Part model, mm, in its own coordinate system. Give positions to 0.01 mm unless a question says otherwise; leave off trailing zeros. Order: outer loops, then holes, each group sorted by start corner. A loop starts at its lowest first (then second) coordinate and runs counter-clockwise, first axis right, second up. Notation, with made-up numbers: M 85,-23 L 93,-23 A18 cw 93,-18 Z; hole C 59.25,9.25 d2. An arc over 180 degrees is marked long. Return JSON: item names as keys, results as strings.
from build123d import *

# Parameters (mm, degrees)
SKETCH1_W           = 49
SKETCH1_H           = 49
SKETCH1_R           = 2
BOSS_EXTRUDE1_DEPTH = 1.6
CHAMFER1_SIZE       = 5
CHAMFER2_SIZE       = 2


with BuildPart() as part:
    # Sketch1 → Boss-Extrude1 (new body)
    with BuildSketch(Plane(origin=(0, 0, 0), x_dir=(0, 1, 0), z_dir=(0, 0, 1))):
        with Locations((24.5, 24.5)):
            Rectangle(SKETCH1_W, SKETCH1_H)
        with Locations(Location((24.5, 26.5, 0), (0, 0, 270))):
            Circle(SKETCH1_R, mode=Mode.SUBTRACT)
    extrude(amount=-BOSS_EXTRUDE1_DEPTH)

    # Chamfer1
    chamfer1_edges = [part.edges().sort_by_distance(p)[0] for p in [
        (-49, 49, -0.8),
    ]]
    chamfer(chamfer1_edges, length=CHAMFER1_SIZE)

    # Chamfer2
    chamfer2_edges = [part.edges().sort_by_distance(p)[0] for p in [
        (-49, 0, -0.8),
        (0, 49, -0.8),
        (0, 0, -0.8),
    ]]
    chamfer(chamfer2_edges, length=CHAMFER2_SIZE)


solid = part.part
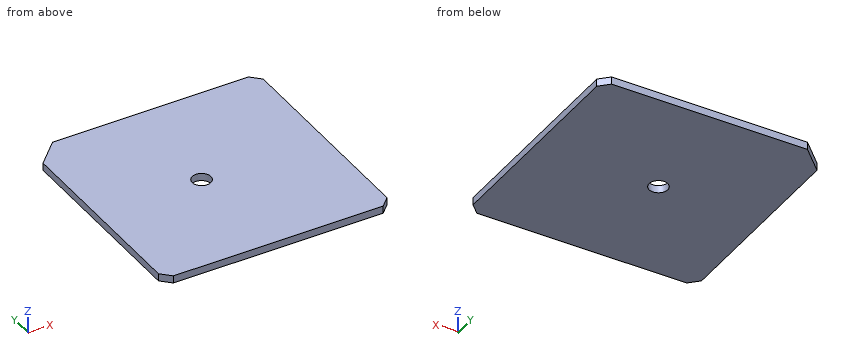
Q1. Pin check, flat tips, straight feed: pin 1 (3.5 mm diameter, centred on x = -26.5, y = 24.5, fed in from -Z); pin 2 (2 mm diameter, centred on x = -43, y = 42, fed in from +Z). Stop position of each tip, or through.
Established:
{"pin 1": "passes through", "pin 2": "stops at z = 0"}
Q2. Band-saw the part on B-B (y = 24.5). Give the cut face in (x, z).
Established:
{"outline": "M -49,-1.6 L -28.5,-1.6 L -28.5,0 L -49,0 Z; M -24.5,-1.6 L 0,-1.6 L 0,0 L -24.5,0 Z"}
Q3. Band-saw the part on A-A (x = -26.5). Give the cut face in (y, z).
Established:
{"outline": "M 0,-1.6 L 22.5,-1.6 L 22.5,0 L 0,0 Z; M 26.5,-1.6 L 49,-1.6 L 49,0 L 26.5,0 Z"}
Q4. Probe line 1 along Y through (x, z) = (-26.5, -1.15); line 2 along X through (y, z) = (46, -0.2); line 3 along X through (y, z) = (25.5, -1). List the from-to ranges inside material, lowest first.
Established:
{"line 1": "y = 0 to 22.5, 26.5 to 49", "line 2": "x = -47 to 0", "line 3": "x = -49 to -28.23, -24.77 to 0"}
